```python
from build123d import *

# Parameters (mm, degrees)
BOSS_EXTRUDE2_DEPTH = 6
SKETCH9_R           = 1.5
CUT_EXTRUDE1_DEPTH  = 7
SKETCH10_W          = 10
SKETCH10_H          = 60
BOSS_EXTRUDE3_DEPTH = 125
SKETCH11_R          = 20
CUT_EXTRUDE2_DEPTH  = 288.855715857


with BuildPart() as part:
    # Sketch8 → Boss-Extrude2 (new body)
    with BuildSketch(Plane(origin=(0, 0, 0), x_dir=(1, 0, 0), z_dir=(0, 1, 0))):
        Polygon((-20, 190.358983854), (20, 190.358983854), (174.855715857, -77.858983852), (154.855715857, -112.500000003), (-154.855715857, -112.500000003), (-174.855715857, -77.858983852), align=None)
    extrude(amount=BOSS_EXTRUDE2_DEPTH)

    # Sketch9 → Cut-Extrude1 (cut, through all)
    with BuildSketch(Plane(origin=(0, 6, 0), x_dir=(1, 0, 0), z_dir=(0, 1, 0))):
        with Locations((15, 185.358983854)):
            Circle(SKETCH9_R)
        with Locations((-15, 185.358983854)):
            Circle(SKETCH9_R)
        with Locations((-15, 179.358983854)):
            Circle(SKETCH9_R)
        with Locations((-15, 173.358983854)):
            Circle(SKETCH9_R)
        with Locations((15, 179.358983854)):
            Circle(SKETCH9_R)
        with Locations((15, 173.358983854)):
            Circle(SKETCH9_R)
        with Locations((153.025588838, -105.669872984)):
            Circle(SKETCH9_R)
        with Locations((168.025588838, -79.68911087)):
            Circle(SKETCH9_R)
        with Locations((162.829436415, -76.68911087)):
            Circle(SKETCH9_R)
        with Locations((157.633283992, -73.68911087)):
            Circle(SKETCH9_R)
        with Locations((147.829436415, -102.669872984)):
            Circle(SKETCH9_R)
        with Locations((142.633283992, -99.669872984)):
            Circle(SKETCH9_R)
        with Locations((-168.025588838, -79.68911087)):
            Circle(SKETCH9_R)
        with Locations((-153.025588838, -105.669872984)):
            Circle(SKETCH9_R)
        with Locations((-147.829436415, -102.669872984)):
            Circle(SKETCH9_R)
        with Locations((-142.633283992, -99.669872984)):
            Circle(SKETCH9_R)
        with Locations((-162.829436415, -76.68911087)):
            Circle(SKETCH9_R)
        with Locations((-157.633283992, -73.68911087)):
            Circle(SKETCH9_R)
    extrude(amount=-CUT_EXTRUDE1_DEPTH, mode=Mode.SUBTRACT)

    # Sketch10 → Boss-Extrude3 (add)
    with BuildSketch(Plane(origin=(0, 6, 0), x_dir=(1, 0, 0), z_dir=(0, 1, 0))):
        with Locations((-108, -36.54767864)):
            Rectangle(SKETCH10_W, SKETCH10_H)
        with Locations((108, -36.54767864)):
            Rectangle(SKETCH10_W, SKETCH10_H)
    extrude(amount=BOSS_EXTRUDE3_DEPTH)

    # Sketch11 → Cut-Extrude2 (cut, through all)
    with BuildSketch(Plane(origin=(113, 0, 0), x_dir=(0, 0, -1), z_dir=(1, 0, 0))):
        with Locations((-36.54767864, 80)):
            Circle(SKETCH11_R)
    extrude(amount=-CUT_EXTRUDE2_DEPTH, mode=Mode.SUBTRACT)


solid = part.part
```
Here's how the part is built. I have some questions about the finished solid (model axes, mm). A direction names the side the tool comes from. Coordinates: 2 decimals unless noted, no trailing zeros. Order: outer loops, then holes, each group sorted by start corner. A loop starts at its lowest first (then second) coordinate and runs counter-clockwise, first axis right, second up.
Item 1: If we section it at B-B, the plane x = -5: List the corners of the cut face in (y, z) for me.
Response values:
outline: (0, -190.36) - (6, -190.36) - (6, 112.5) - (0, 112.5) - close
Item 2: Thinking about a two-plate mould opening in X: for faces 1 (the face through (-108, 131, 36)), 2 (the face through (-103, 54, 37)), 3 (the face through (103, 54, 37)), 4 (the face through (-164.716, 2.958, 95.422)), which applies, pulls with the +X half, pulls with the -X half, needs draft (parallel to the pull), parting line crosses it, or undercut?
Response values:
face 1: needs draft
face 2: undercut
face 3: undercut
face 4: pulls with the -X half
Item 3: Which directions (+Z, -Z, +X, -X, +Y, -Y) give clear straight access to the entire face, cutting with the end or side of a thin tool? Please do faces 5 (the face through (108, 68, 6.548)), 6 (the face through (-108, 68, 66.548)), 7 (the face through (113, 54, 37)).
Response values:
face 5: -Z, +X, -X, +Y
face 6: +Z, +X, -X, +Y
face 7: +Z, -Z, +X, +Y
Item 4: If we section it at A-A, the plane y = 80: List the corners of the cut face in (x, z) for me.
Response values:
outline: (-113, 6.55) - (-103, 6.55) - (-103, 16.55) - (-113, 16.55) - close; (-113, 56.55) - (-103, 56.55) - (-103, 66.55) - (-113, 66.55) - close; (103, 6.55) - (113, 6.55) - (113, 16.55) - (103, 16.55) - close; (103, 56.55) - (113, 56.55) - (113, 66.55) - (103, 66.55) - close
Item 5: If we section it at C-C, the plane z = 11.5: List the corners of the cut face in (x, y) for me.
Response values:
outline: (-136.54, 0) - (136.54, 0) - (136.54, 6) - (113, 6) - (113, 131) - (103, 131) - (103, 6) - (-103, 6) - (-103, 131) - (-113, 131) - (-113, 6) - (-136.54, 6) - close
Item 6: I need wall thicknesses on probe 1 along X at (y, z) = (84.5, 64); probe 2 along Y at (x, z) = (74, 9). Which ranges of each line are inside material? Lowest first, please.
Response values:
probe 1: x = -113 to -103, 103 to 113
probe 2: y = 0 to 6
Item 7: I'm going to push flat-ended pins straight in: pin 1 Ø2.5 at (x, z) = (147.83, 102.67) entering from +Y; pin 2 Ø5 at (x, z) = (15, -173.36) entering from -Y; pin 3 Ø11 at (x, y) = (106.5, 80.5) entering from -Z; pin 4 Ø5 at (x, z) = (-162.83, 76.69) entering from +Y. Where does each tip first touch, or does it pass through?
Response values:
pin 1: passes through
pin 2: stops at y = 0
pin 3: stops at z = 6.55
pin 4: stops at y = 6
Item 8: If we section it at D-D, the plane x = -53: List the corners of the cut face in (y, z) for me.
Response values:
outline: (0, -133.2) - (6, -133.2) - (6, 112.5) - (0, 112.5) - close
